from build123d import *

# Parameters (mm, degrees)
CROQUIS1_R              = 18
CROQUIS1_R_2            = 9.1
SALIENTE_EXTRUIR1_DEPTH = 7
CROQUIS2_R              = 14.75
CROQUIS2_R_2            = 11.2
CORTAR_EXTRUIR1_DEPTH   = 3
CHAFL_N1_SIZE           = 0.5


with BuildPart() as part:
    # Croquis1 → Saliente-Extruir1 (new body)
    with BuildSketch(Plane.XY):
        Circle(CROQUIS1_R)
        Circle(CROQUIS1_R_2, mode=Mode.SUBTRACT)
    extrude(amount=SALIENTE_EXTRUIR1_DEPTH)

    # Croquis2 → Cortar-Extruir1 (cut)
    with BuildSketch(Plane.XY.offset(7)):
        Circle(CROQUIS2_R)
        Circle(CROQUIS2_R_2, mode=Mode.SUBTRACT)
    extrude(amount=-CORTAR_EXTRUIR1_DEPTH, mode=Mode.SUBTRACT)

    # Chaflán1
    chafl_n1_edges = [part.edges().sort_by_distance(p)[0] for p in [
        (-14.75, 0, 7),
        (-11.2, 0, 7),
        (-18, 0, 0),
        (-18, 0, 7),
        (-9.1, 0, 0),
        (-9.1, 0, 7),
    ]]
    chamfer(chafl_n1_edges, length=CHAFL_N1_SIZE)


solid = part.part
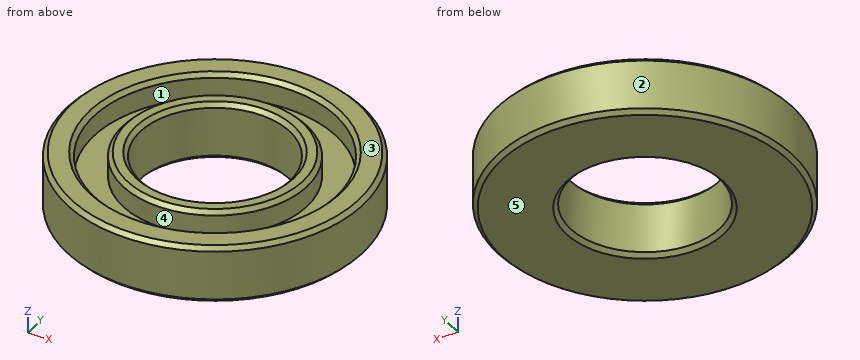
CAD build for the part. Positions are in the model's coordinates, mm. Face numbers are marked on the shaded views. A direction names the side the tool comes from. Give positions to 0.01 mm unless a question says otherwise; leave off trailing zeros. Loops run counter-clockwise (first coordinate to the right, second up) from the corner with the lowest first, then second, coordinate; pieces in that order, holes last. Notation, with made-up numbers: M 42.5,-33 L 73.5,-33 A25 cw 73.5,-10 Z; hole C 84.5,46 d6. An arc over 180 degrees is marked long. Write each question's results on one line, items separated by ' | '.
Q1. Band-saw the part on B-B on z = 5. Write the cut outline in (x, y).
Geometry check:
outline: C 0,0 d36; C 0,0 d22.4; hole C 0,0 d29.5; hole C 0,0 d18.2
Q2. Band-saw the part on A-A on x = 0. Write the cut outline in (y, z).
Geometry check:
outline: M -18,0.5 L -17.5,0 L -9.6,0 L -9.1,0.5 L -9.1,6.5 L -9.6,7 L -10.7,7 L -11.2,6.5 L -11.2,4 L -14.75,4 L -14.75,6.5 L -15.25,7 L -17.5,7 L -18,6.5 Z; M 9.1,0.5 L 9.6,0 L 17.5,0 L 18,0.5 L 18,6.5 L 17.5,7 L 15.25,7 L 14.75,6.5 L 14.75,4 L 11.2,4 L 11.2,6.5 L 10.7,7 L 9.6,7 L 9.1,6.5 Z
Q3. Band-saw the part on D-D on z = 2.5. Write the cut outline in (x, y), and give its area (3 significant figures).
Geometry check:
outline: C 0,0 d36; hole C 0,0 d18.2 | area: 758 mm²
Q4. Which spindle directions (+Z, -Z, +X, -X, +Y, -Y) get a long thin tool onto all of the face, cutting with end or side? Do the marked faces 4 and 5. Say none if no direction does.
Geometry check:
face 4: +Z | face 5: -Z, +X, -X, +Y, -Y
Q5. Probe probe 1 along Y at (x, z) = (0, 4.7); probe 2 along Y at (x, z) = (-6, 5.5); probe 3 along X at (y, z) = (-0.5, 6). List the from-to ranges inside material, lowest first.
Geometry check:
probe 1: y = -18 to -14.75, -11.2 to -9.1, 9.1 to 11.2, 14.75 to 18 | probe 2: y = -16.97 to -13.47, -9.46 to -6.84, 6.84 to 9.46, 13.47 to 16.97 | probe 3: x = -17.99 to -14.74, -11.19 to -9.09, 9.09 to 11.19, 14.74 to 17.99
Q6. Flat gauge pins, fed straight in: P1, Ø1, axis at x = -10, z = 3.5, coming from the +Y side; P2, Ø1, axis at y = -8, z = 3, coming from the +X side; P3, Ø12, axis at x = -11.5, y = 8.5, coming from the -Z side; P4, Ø2, axis at y = 3.5, z = 1, coming from the +X side. Where does each tip first touch, or does it go through?
Geometry check:
P1: stops at y = 15.29 | P2: stops at x = 16.36 | P3: stops at z = 0 | P4: stops at x = 17.83
Q7. Mould opens along Y. For the marked faces 1, 2 and 3 say: pulls with the +Y half, pulls with the -Y half, needs draft (parallel to the pull), parting line crosses it, or undercut.
Geometry check:
face 1: undercut | face 2: parting line crosses it | face 3: needs draft
